For this review, use the dimensioned drawing (mm, ordinates from the lowest corner) and the shaded views. Coordinates: 2 decimals unless noted, no trailing zeros. Loops run counter-clockwise (first coordinate to the right, second up) from the corner with the lowest first, then second, coordinate; pieces in that order, holes last. Notation, with made-up numbers: (73.5, 60.25) -> (130.5, 60.25) arc R17 cw to (130.5, 74.25) -> close; hole circle Ø11 at (-18.5, 42). An arc over 180 degrees is marked (long way). Answer as a JSON object with one key per item and string values.
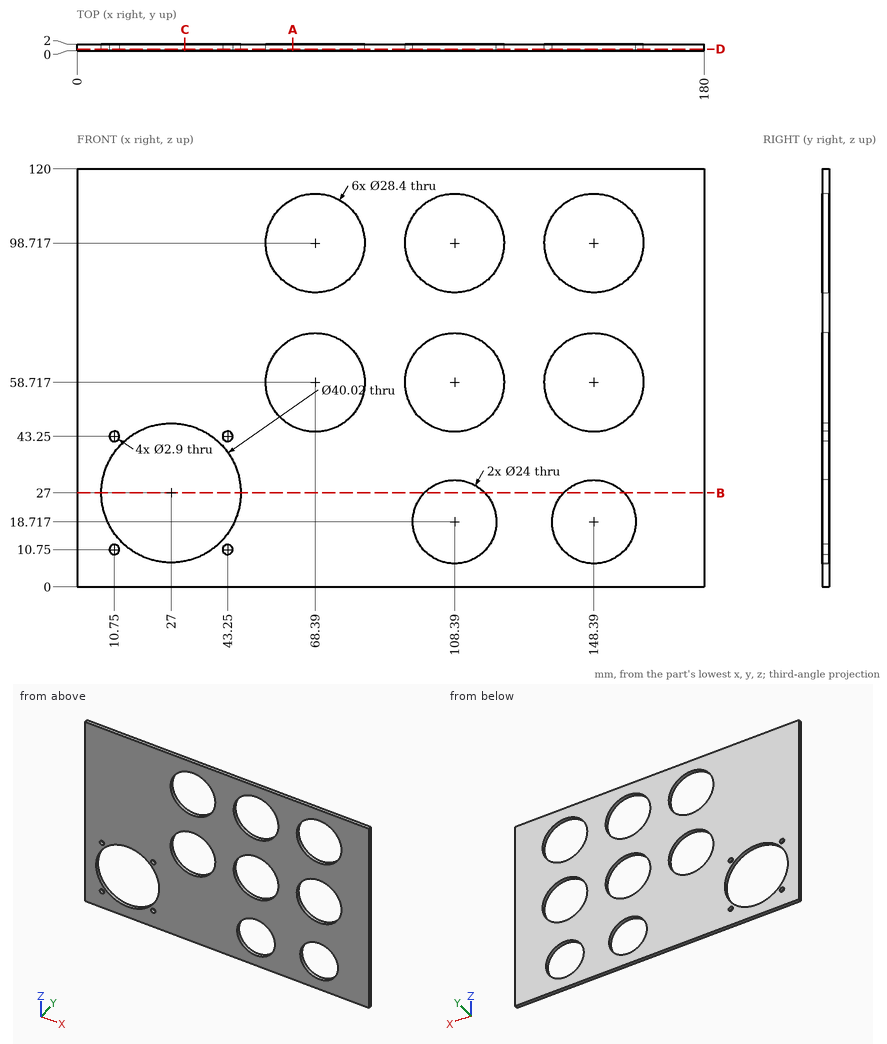
1) Add section B-B, the plane z = 27. Give the boundary of the cut face in (x, y).
Completed:
{"outline": "(0, 0) -> (6.99, 0) -> (6.99, 2) -> (0, 2) -> close; (47.01, 0) -> (99.71, 0) -> (99.71, 2) -> (47.01, 2) -> close; (117.07, 0) -> (139.71, 0) -> (139.71, 2) -> (117.07, 2) -> close; (157.07, 0) -> (180, 0) -> (180, 2) -> (157.07, 2) -> close"}
2) Add section C-C, the plane x = 31. Give the boundary of the cut face in (y, z).
Completed:
{"outline": "(0, 0) -> (2, 0) -> (2, 7.39) -> (0, 7.39) -> close; (0, 46.61) -> (2, 46.61) -> (2, 120) -> (0, 120) -> close"}
3) Add section D-D, the plane y = 0.55. Count the separate pieces of the cut face and the enclosed holes in it, and give its area (3 significant figures).
Completed:
{"separate pieces": "1", "enclosed holes": "13", "area": "15,600 mm²"}
4) Wall thickness on probe 1 along X at (y, z) = (0.5, 98.5); probe 2 along Z at (x, y) = (154, 1.6) (1 decimal); probe 3 along Z at (x, y) = (43.25, 0.5) (1 decimal): over which ranges is each line inside the solid? List them lowest first.
Completed:
{"probe 1": "0 to 54.19, 82.59 to 94.19, 122.59 to 134.19, 162.59 to 180", "probe 2": "0 to 8.1, 29.3 to 45.7, 71.8 to 85.7, 111.8 to 120", "probe 3": "0 to 9.3, 12.2 to 15.3, 38.7 to 41.8, 44.7 to 120"}
5) Add section A-A, the plane x = 62. Give the boundary of the cut face in (y, z).
Completed:
{"outline": "(0, 0) -> (2, 0) -> (2, 46.04) -> (0, 46.04) -> close; (0, 71.4) -> (2, 71.4) -> (2, 86.04) -> (0, 86.04) -> close; (0, 111.4) -> (2, 111.4) -> (2, 120) -> (0, 120) -> close"}
